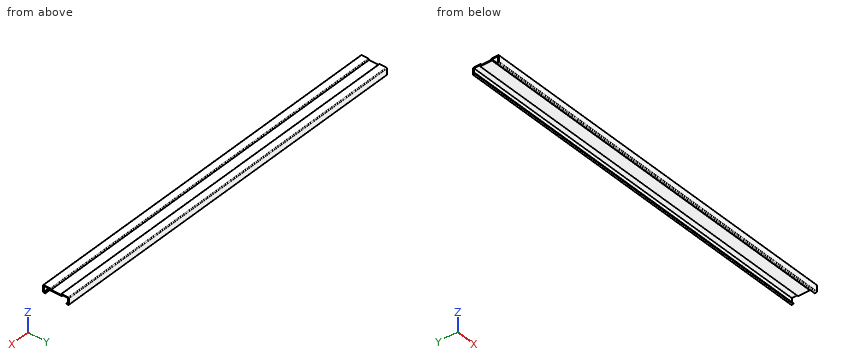
```python
from build123d import *

# Parameters (mm, degrees)
EXTRUDE_3_DEPTH = 500


with BuildPart() as part:
    # Эскиз1 → Вытянуть-Тонкостенный3 (new body)
    with BuildSketch(Plane(origin=(0, 0, 0), x_dir=(0, 0, -1), z_dir=(1, 0, 0))):
        with BuildLine():
            Line((8, 14), (8, 16))
            ThreePointArc((8, 16), (7.707106781, 16.707106781), (7, 17))
            Line((7, 17), (-0.5, 17))
            ThreePointArc((-0.5, 17), (-1.207106781, 16.707106781), (-1.5, 16))
            Line((-1.5, 16), (-1.5, 7.5))
            ThreePointArc((-1.5, 7.5), (-1.207106781, 6.792893219), (-0.5, 6.5))
            Line((-0.5, 6.5), (0, 6.5))
            Line((0, 6.5), (0, -6.5))
            Line((0, -6.5), (-0.5, -6.5))
            ThreePointArc((-0.5, -6.5), (-1.207106781, -6.792893219), (-1.5, -7.5))
            Line((-1.5, -7.5), (-1.5, -16))
            ThreePointArc((-1.5, -16), (-1.207106781, -16.707106781), (-0.5, -17))
            Line((-0.5, -17), (7, -17))
            ThreePointArc((7, -17), (7.707106781, -16.707106781), (8, -16))
            Line((8, -16), (8, -14))
            Line((8, -14), (6.8, -14))
            Line((6.8, -14), (6.8, -15.8))
            Line((6.8, -15.8), (-0.3, -15.8))
            Line((-0.3, -15.8), (-0.3, -7.7))
            Line((-0.3, -7.7), (1.2, -7.7))
            Line((1.2, -7.7), (1.2, 7.7))
            Line((1.2, 7.7), (-0.3, 7.7))
            Line((-0.3, 7.7), (-0.3, 15.8))
            Line((-0.3, 15.8), (6.8, 15.8))
            Line((6.8, 15.8), (6.8, 14))
            Line((6.8, 14), (8, 14))
        make_face()
    extrude(amount=EXTRUDE_3_DEPTH)


solid = part.part
```
Check sheet for the modelled part. Datum: model origin and axes. Units: mm. Round coordinates to 2 decimals unless told otherwise and drop trailing zeros. Order: outer loops, then holes, each group sorted by start corner. A loop starts at its lowest first (then second) coordinate and runs counter-clockwise, first axis right, second up. Notation, with made-up numbers: (-35.75, 44.25) - (8.25, 44.25) arc R21 ccw to (8.25, 64.25) - close; hole circle Ø3 at (2.5, 26.5). An arc over 180 degrees is marked (long way). Write item = value, one per line.
Q1. Section check B-B (x = 230.5). Record the boundary of the cut face in (y, z).
Computed:
outline = (-17, -7) arc R1 ccw to (-16, -8) - (-14, -8) - (-14, -6.8) - (-15.8, -6.8) - (-15.8, 0.3) - (-7.7, 0.3) - (-7.7, -1.2) - (7.7, -1.2) - (7.7, 0.3) - (15.8, 0.3) - (15.8, -6.8) - (14, -6.8) - (14, -8) - (16, -8) arc R1 ccw to (17, -7) - (17, 0.5) arc R1 ccw to (16, 1.5) - (7.5, 1.5) arc R1 ccw to (6.5, 0.5) - (6.5, 0) - (-6.5, 0) - (-6.5, 0.5) arc R1 ccw to (-7.5, 1.5) - (-16, 1.5) arc R1 ccw to (-17, 0.5) - close
Q2. Thickness scan on line 1 along Y through (x, z) = (53, -0.5); line 2 along Y through (x, z) = (81, -4.75); line 3 along Z through (x, y) = (67.5, -8.5). Record the ranges inside material, lowest first.
Computed:
line_1 = -17 to -15.8, -7.7 to 7.7, 15.8 to 17
line_2 = -17 to -15.8, 15.8 to 17
line_3 = 0.3 to 1.5
Q3. Section check C-C (y = 1). Record the boundary of the cut face in (x, z).
Computed:
outline = (0, -1.2) - (500, -1.2) - (500, 0) - (0, 0) - close
Q4. Section check A-A (z = -4). Record the boundary of the cut face in (x, y), and give its area (3 significant figures).
Computed:
outline = (0, -17) - (500, -17) - (500, -15.8) - (0, -15.8) - close; (0, 15.8) - (500, 15.8) - (500, 17) - (0, 17) - close
area = 1,200 mm^2
Q5. Go/stop test with flat-tipped pins: pin 1 (2.5 mm diameter, centred on x = 341.5, y = -10.5, fed in from -Z); pin 2 (12 mm diameter, centred on x = 257.5, y = 7.5, fed in from -Z); pin 3 (0.6 mm diameter, centred on x = 370, z = -7.5, fed in from -Y). Record where each tip stops, or that it passes through.
Computed:
pin_1 = 0.3
pin_2 = -1.2
pin_3 = -16.98
